```python
from build123d import *

# Parameters (mm, degrees)
SKETCH1_W           = 304.8
SKETCH1_H           = 12.7
BOSS_EXTRUDE1_DEPTH = 6.35


with BuildPart() as part:
    # Sketch1 → Boss-Extrude1 (new body)
    with BuildSketch(Plane.XY):
        Rectangle(SKETCH1_W, SKETCH1_H)
        with BuildLine():
            ThreePointArc((-146.05, -1.27), (-147.32, 0), (-146.05, 1.27))
            Line((-146.05, 1.27), (146.05, 1.27))
            ThreePointArc((146.05, 1.27), (146.948025612, 0.898025612), (147.32, 0))
            ThreePointArc((147.32, 0), (146.948025612, -0.898025612), (146.05, -1.27))
            Line((146.05, -1.27), (-146.05, -1.27))
        make_face(mode=Mode.SUBTRACT)
    extrude(amount=BOSS_EXTRUDE1_DEPTH)


solid = part.part
```
Work out the finished part from the listing and answer in its coordinate system (mm). A direction names the side the tool comes from. Round coordinates to 2 decimals unless told otherwise and drop trailing zeros. Loops run counter-clockwise (first coordinate to the right, second up) from the corner with the lowest first, then second, coordinate; pieces in that order, holes last. Notation, with made-up numbers: M 77.5,-16.5 L 117.5,-16.5 A28 cw 117.5,19.5 Z; hole C 5,17.5 d8. An arc over 180 degrees is marked long. Use CSV: the item, a comma, the result in double quotes.
Q1. This flat-tipped pin is pushed along its axis until it touches: pin 1 (6 mm diameter, centred on x = -54.5, y = -4, fed in from -Z). Where does it stop, or does it pass through?
Determined:
pin 1,"z = 0"
Q2. Consider L1, parallel to Y at x = 74, z = 3.25. Determine where the line is inside the solid, lowest interval first.
Determined:
L1,"-6.35 to -1.27, 1.27 to 6.35"
Q3. Section A-A, the plane x = -76 is taken. Determine the outline of the cut face in (y, z), then the cut area to 3 significant figures.
Determined:
outline,"M -6.35,0 L -1.27,0 L -1.27,6.35 L -6.35,6.35 Z; M 1.27,0 L 6.35,0 L 6.35,6.35 L 1.27,6.35 Z"
area,"64.5 mm2"
Q4. The mould has two halves that part along Y. Classify faces 1 (the flat face through (-2, 6.35, 3)), 2 (the flat face through (-2, -6.35, 3)), 3 (the flat face through (-2, 1.27, 3)): pulls with the +Y half, pulls with the -Y half, needs draft (parallel to the pull), parting line crosses it, or undercut.
Determined:
face 1,"pulls with the +Y half"
face 2,"pulls with the -Y half"
face 3,"undercut"
Q5. A tool of negligible diameter and unlimited length cuts with its end or side. For faces 4 (the flat face through (-2, 2, 0)), 5 (the flat face through (2, -1.27, 3)), from which of +Z, -Z, +X, -X, +Y, -Y can it reach the whole face along a straight path? Write none if from no direction.
Determined:
face 4,"-Z, +X, -X, +Y, -Y"
face 5,"+Z, -Z"
Q6. Section B-B, the plane z = 5 is taken. Determine the outline of the cut face in (x, y), then the cut area to 3 significant figures.
Determined:
outline,"M -152.4,-6.35 L 152.4,-6.35 L 152.4,6.35 L -152.4,6.35 Z; hole M -146.05,-1.27 L 146.05,-1.27 A1.27 ccw 146.05,1.27 L -146.05,1.27 A1.27 ccw Z"
area,"3,120 mm2"
